Here's how the part is built. I have some questions about the finished solid (model axes, mm). Coordinates: 2 decimals unless noted, no trailing zeros. Write each loop counter-clockwise with the first axis right and the second up, starting at its lowest first coordinate (ties: lowest second). Pieces come first, ordered by that corner, then holes. Notation, with made-up numbers: M 19,-24.5 L 53,-24.5 A7 cw 53,-17.5 Z; hole C -12,12.25 d4. An arc over 180 degrees is marked long. Use one line per item in the form item = value. Start each with the question number.
1. I want a section at B-B, the plane x = 27. List the corners of the cut face in (y, z) for me, plus the area to 3 significant figures.
2. Please list where these lines run through material, in increasing order: line 1 along X through (y, z) = (-31.5, 0.75); line 2 along Y through (x, z) = (-22, 2.1); line 3 along X through (y, z) = (-29, 2.6). Write a range as [from, to].
3. I want a section at C-C, the plane y = 35. List the corners of the cut face in (x, z) for me.
4. I'm going to push flat-ended pins straight in: pin 1 Ø1.5 at (y, z) = (19.5, 0.5) entering from -X; pin 2 Ø2 at (y, z) = (-48.5, 2) entering from -X. Where does each tip first touch, or does it pass through?
5. I want a section at A-A, the plane z = 1.45. List the corners of the cut face in (x, y) for me.
from build123d import *

# Parameters (mm, degrees)
BOSS_EXTRUDE1_DEPTH = 4.3


with BuildPart() as part:
    # Sketch3 → Boss-Extrude1 (new body)
    with BuildSketch(Plane.XY):
        with BuildLine():
            Line((-20, 47.7), (20, 47.7))
            ThreePointArc((20, 47.7), (41.708178182, 38.708178182), (50.7, 17))
            Line((50.7, 17), (50.7, -28))
            ThreePointArc((50.7, -28), (40.243712088, -53.243712088), (15, -63.7))
            Line((15, -63.7), (0.5, -63.7))
            Line((0.5, -63.7), (-0.5, -63.7))
            Line((-0.5, -63.7), (-15, -63.7))
            ThreePointArc((-15, -63.7), (-40.243712088, -53.243712088), (-50.7, -28))
            Line((-50.7, -28), (-50.7, 17))
            ThreePointArc((-50.7, 17), (-41.708178182, 38.708178182), (-20, 47.7))
        make_face()
    extrude(amount=BOSS_EXTRUDE1_DEPTH)


solid = part.part
Answer list:
q1.outline = M -61.62,0 L 46.89,0 L 46.89,4.3 L -61.62,4.3 Z
q1.area = 467 mm²
q2.line_1 = [-50.53, 50.53]
q2.line_2 = [-63.01, 47.63]
q2.line_3 = [-50.69, 50.69]
q3.outline = M -44.87,0 L 44.87,0 L 44.87,4.3 L -44.87,4.3 Z
q4.pin_1 = -50.65
q4.pin_2 = -44.9
q5.outline = M -50.7,-28 A35.7 ccw -15,-63.7 L 15,-63.7 A35.7 ccw 50.7,-28 L 50.7,17 A30.7 ccw 20,47.7 L -20,47.7 A30.7 ccw -50.7,17 Z
